The drawing under review shows one solid part. Ordinate dimensions are in mm from its lowest x, y, z. Round coordinates to 2 decimals unless told otherwise and drop trailing zeros. Write each loop counter-clockwise with the first axis right and the second up, starting at its lowest first coordinate (ties: lowest second). Pieces come first, ordered by that corner, then holes.
Item 1: To check wall thickness, follow L1, parallel to Z at x = 7.5, y = 8.89; L2, parallel to Y at x = 11.25, z = 10; L3, parallel to Z at x = 22.5, y = 9.25 (1 decimal). State the ranges of each line that lie inside material, in increasing order.
Item 2: Draft analysis for pull direction Z (two halves, no side actions). For the marked faces 1, 2 and 3, state which applies: +Z half, -Z half, draft (parallel to the pull), parting line (faces both ways), or undercut.
Item 3: Add section A-A (y = 8.89). Give the boundary of the cut face in (x, z).
Item 4: Add section B-B (z = 7.75). Give the boundary of the cut face in (x, y).
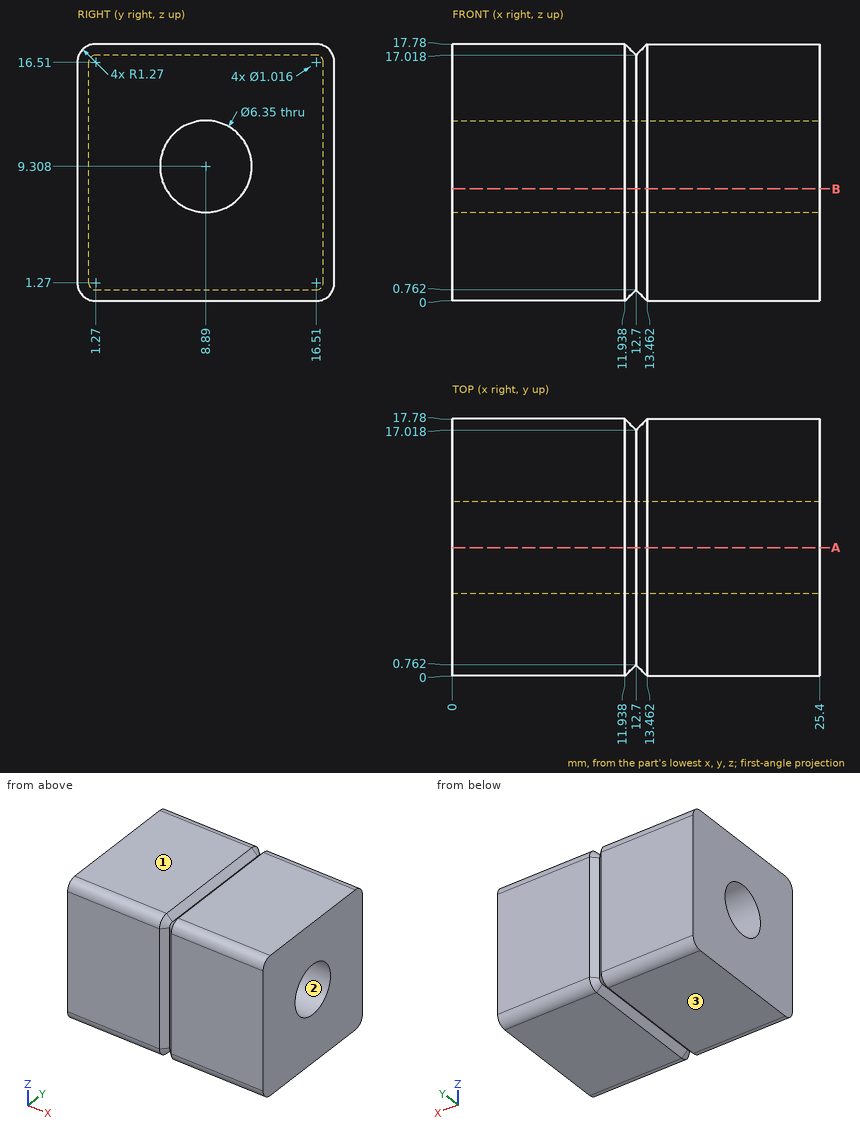
Numbers:
1. L1: z = 0 to 6.13, 12.48 to 17.78
1. L2: y = 0 to 5.79, 11.99 to 17.78
1. L3: z = 0 to 6.2, 12.5 to 17.8
2. face 1: +Z half
2. face 2: undercut
2. face 3: -Z half
3. outline: (0, 0) - (11.94, 0) - (12.7, 0.76) - (13.46, 0) - (25.4, 0) - (25.4, 6.13) - (0, 6.13) - close; (0, 12.48) - (25.4, 12.48) - (25.4, 17.78) - (13.46, 17.78) - (12.7, 17.02) - (11.94, 17.78) - (0, 17.78) - close
4. outline: (0, 0) - (11.94, 0) - (12.7, 0.76) - (13.46, 0) - (25.4, 0) - (25.4, 6.12) - (0, 6.12) - close; (0, 11.66) - (25.4, 11.66) - (25.4, 17.78) - (13.46, 17.78) - (12.7, 17.02) - (11.94, 17.78) - (0, 17.78) - close
